Verification items for the finished model (mm, model axes). A direction names the side the tool comes from. Round coordinates to 2 decimals unless told otherwise and drop trailing zeros. Write each loop counter-clockwise with the first axis right and the second up, starting at its lowest first coordinate (ties: lowest second). Pieces come first, ordered by that corner, then holes. Notation, with made-up numbers: (-3, 22) - (41, 22) arc R19 cw to (41, 59) - close; hole circle Ø8 at (-13.75, 66). An arc over 180 degrees is marked (long way). Answer as a JSON object with one key per item and string values.
```python
from build123d import *

# Parameters (mm, degrees)
F0_W     = 38.1
F0_H     = 25.4
F1_DEPTH = 25.4
F3_W     = 6.35
F3_H     = 7.8098609388
F4_DEPTH = 38.101
F5_W     = 6.35
F5_H     = 6.35
F6_DEPTH = 25.401


with BuildPart() as f1:
    # F0 (on Front) → F1 (new body)
    with BuildSketch(Plane.XZ):
        with Locations((-19.05, 12.7)):
            Rectangle(F0_W, F0_H)
    extrude(amount=F1_DEPTH)

    # F3 (on face) → F4 (cut, through all)
    with BuildSketch(Plane(origin=(-38.1, 0, 0), x_dir=(0, -1, 0), z_dir=(-1, 0, 0))):
        with Locations((10.7136315584, 21.4950695306)):
            Rectangle(F3_W, F3_H)
    extrude(amount=-F4_DEPTH, mode=Mode.SUBTRACT)

    # F5 (on face) → F6 (cut, through all)
    with BuildSketch(Plane.XZ.offset(25.4)):
        with Locations((-20.6470728934, 3.175)):
            Rectangle(F5_W, F5_H)
    extrude(amount=-F6_DEPTH, mode=Mode.SUBTRACT)


solid = f1.part
```
Q1. Section check B-B, the plane x = -5.5. Record the cut outline in (y, z).
Geometry check:
{"outline": "(-25.4, 0) - (0, 0) - (0, 25.4) - (-7.54, 25.4) - (-7.54, 17.59) - (-13.89, 17.59) - (-13.89, 25.4) - (-25.4, 25.4) - close"}
Q2. Material ranges on line 1 along X through (y, z) = (-3.75, 3); line 2 along Z through (x, y) = (-18.5, -19); line 3 along Z through (x, y) = (-34, -9.25), recorded low to high. Write a range as [from, to].
Geometry check:
{"line 1": "x = [-38.1, -23.82], [-17.47, 0]", "line 2": "z = [6.35, 25.4]", "line 3": "z = [0, 17.59]"}
Q3. Release check for a two-part mould opening along Y. For faces 1 (the flat face through (-23.822, -13, 3)), 2 (the flat face through (-19, 0, 13)), 3 (the flat face through (-19, -11, 17.59)) record: released by +Y, released by -Y, zero draft, split by the parting line, or undercut.
Geometry check:
{"face 1": "zero draft", "face 2": "released by +Y", "face 3": "undercut"}
Q4. Section check D-D, the plane z = 20.5. Record the cut outline in (x, y), then the cut area to 3 significant figures.
Geometry check:
{"outline": "(-38.1, -25.4) - (0, -25.4) - (0, -13.89) - (-38.1, -13.89) - close; (-38.1, -7.54) - (0, -7.54) - (0, 0) - (-38.1, 0) - close", "area": "726 mm2"}
Q5. Section check A-A, the plane z = 2.75. Record the cut outline in (x, y), then the cut area to 3 significant figures.
Geometry check:
{"outline": "(-38.1, -25.4) - (-23.82, -25.4) - (-23.82, 0) - (-38.1, 0) - close; (-17.47, -25.4) - (0, -25.4) - (0, 0) - (-17.47, 0) - close", "area": "806 mm2"}
Q6. Set-up check for faces 4 (the flat face through (-21, -13, 6.35)), 5 (the flat face through (-19, -7.539, 21)), 6 (the flat face through (-38.1, -13, 13)): record each of +Z, -Z, +X, -X, +Y, -Y from which the full face is reachable in a straight line by a thin tool's end or side.
Geometry check:
{"face 4": "-Z, +Y, -Y", "face 5": "+Z, +X, -X", "face 6": "+Z, -Z, -X, +Y, -Y"}
Q7. Section check C-C, the plane y = -5.5. Record the cut outline in (x, z), then the cut area to 3 significant figures.
Geometry check:
{"outline": "(-38.1, 0) - (-23.82, 0) - (-23.82, 6.35) - (-17.47, 6.35) - (-17.47, 0) - (0, 0) - (0, 25.4) - (-38.1, 25.4) - close", "area": "927 mm2"}
Q8. Gauge pin test, flat ends, axial feed: P1, Ø2, axis at y = -11.5, z = 12.5, coming from the +X side; P2, Ø1.9, axis at x = -15, y = -9, coming from the +Z side. Record the tip position at first contact, or that the pin passes through.
Geometry check:
{"P1": "stops at x = 0", "P2": "stops at z = 17.59"}
